Source: CAD feature listing. Evaluate the final solid. Frame: model axes, mm. Face numbers are marked on the shaded views. A direction names the side the tool comes from. Give positions to 0.01 mm unless a question says otherwise; leave off trailing zeros. Order: outer loops, then holes, each group sorted by start corner. A loop starts at its lowest first (then second) coordinate and runs counter-clockwise, first axis right, second up. Notation, with made-up numbers: (47.5, 32.25) - (94.5, 32.25) arc R29 cw to (94.5, 59.25) - close; hole circle Ø3 at (63, 76.5). An arc over 180 degrees is marked (long way). Answer as CSV lines item,"result".
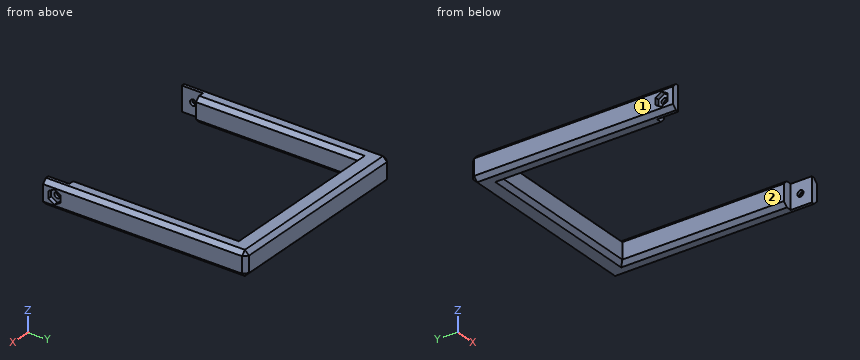
```python
from build123d import *

# Parameters (mm, degrees)
SKETCH1_W             = 3.5
SKETCH1_H             = 12
BOSS_EXTRUDE1_DEPTH   = 100
BOSS_EXTRUDE1_2_DEPTH = 100
SKETCH2_W             = 12
SKETCH2_H             = 10
BOSS_EXTRUDE2_DEPTH   = 90.08829946
SKETCH3_W             = 4.58560389
SKETCH3_H             = 12
BOSS_EXTRUDE3_DEPTH   = 79.6
CHAMFER6_SIZE         = 2
CUT_EXTRUDE1_DEPTH    = 2
CUT_EXTRUDE2_REACH    = 140.122
SKETCH5_R             = 1.5


with BuildPart() as part:
    # Sketch1 → Boss-Extrude1 (new body)
    with BuildSketch(Plane(origin=(0, 0, 0), x_dir=(1, 0, 0), z_dir=(0, 1, 0))):
        with Locations((-46.79414973, 0)):
            Rectangle(SKETCH1_W, SKETCH1_H)
    extrude(amount=BOSS_EXTRUDE1_DEPTH)



with BuildPart() as body_2:
    # Sketch1 → Boss-Extrude1 2 (new body)
    with BuildSketch(Plane(origin=(0, 0, 0), x_dir=(1, 0, 0), z_dir=(0, 1, 0))):
        with Locations((46.79414973, 0)):
            Rectangle(SKETCH1_W, SKETCH1_H)
    extrude(amount=BOSS_EXTRUDE1_2_DEPTH)


with BuildPart() as part_1:
    add(part.part)

    add(body_2.part)  # Boss-Extrude2 merges body 2
    # Sketch2 → Boss-Extrude2 (add)
    with BuildSketch(Plane(origin=(-45.04414973, 0, 0), x_dir=(0, 0, -1), z_dir=(1, 0, 0))):
        with Locations((0, 95)):
            Rectangle(SKETCH2_W, SKETCH2_H)
    extrude(amount=BOSS_EXTRUDE2_DEPTH)

    # Sketch3 → Boss-Extrude3 (add)
    with BuildSketch(Plane.XZ.offset(-90)):
        with Locations((-42.751347785, 0)):
            Rectangle(SKETCH3_W, SKETCH3_H)
        with Locations((42.751347785, 0)):
            Rectangle(SKETCH3_W, SKETCH3_H)
    extrude(amount=BOSS_EXTRUDE3_DEPTH)

    # Chamfer6
    chamfer6_edges = [part_1.edges().sort_by_distance(p)[0] for p in [
        (0, 100, 6),
        (48.54414973, 50, 6),
        (48.54414973, 50, -6),
        (48.54414973, 100, 0),
        (0, 100, -6),
        (-40.45854584, 50.2, -6),
        (-40.45854584, 50.2, 6),
        (0, 90, 6),
        (0, 90, -6),
        (40.45854584, 50.2, 6),
        (40.45854584, 50.2, -6),
        (-48.54414973, 50, 6),
        (-48.54414973, 50, -6),
        (-48.54414973, 100, 0),
    ]]
    chamfer(chamfer6_edges, length=CHAMFER6_SIZE)

    # Sketch4 → Cut-Extrude1 (cut)
    with BuildSketch(Plane(origin=(48.54414973, 0, 0), x_dir=(0, 0, -1), z_dir=(1, 0, 0))):
        Polygon((3.464101615, 5.6), (1.732050808, 8.6), (-1.732050808, 8.6), (-3.464101615, 5.6), (-1.732050808, 2.6), (1.732050808, 2.6), align=None)
    cut_extrude1 = extrude(amount=-CUT_EXTRUDE1_DEPTH, mode=Mode.SUBTRACT)

    # Mirror1: Cut-Extrude1 across plane
    add(cut_extrude1.mirror(Plane(origin=(0, 0, 0), x_dir=(0, 0, 1), z_dir=(1, 0, 0))), mode=Mode.SUBTRACT)

    # Cut-Extrude2: up to this face of the body (flat: up to its plane)
    cut_extrude2_end = Plane(part_1.part.faces().sort_by_distance((-46.54414973, 5.6, 0))[0])
    # Sketch5 → Cut-Extrude2 (cut, up to the picked face)
    with BuildSketch(Plane(origin=(46.54414973, 0, 0), x_dir=(0, 0, -1), z_dir=(1, 0, 0)), mode=Mode.PRIVATE) as cut_extrude2_sk1:
        with Locations((0, 5.6)):
            Circle(SKETCH5_R)
    cut_extrude2_tool1 = split(extrude(cut_extrude2_sk1.sketch, amount=-CUT_EXTRUDE2_REACH, mode=Mode.PRIVATE), bisect_by=cut_extrude2_end, keep=Keep.BOTH, mode=Mode.PRIVATE)
    add(cut_extrude2_tool1.solids().sort_by(Axis((46.54415, 5.6, 0), (-1, 0, 0)))[0], mode=Mode.SUBTRACT)


solid = part_1.part
```
(1) Cut plane B-B (y = 69). Return loops of the section in (x, z).
Completed:
outline,"(-48.54, -4) - (-46.54, -6) - (-42.46, -6) - (-40.46, -4) - (-40.46, 4) - (-42.46, 6) - (-46.54, 6) - (-48.54, 4) - close; (40.46, -4) - (42.46, -6) - (46.54, -6) - (48.54, -4) - (48.54, 4) - (46.54, 6) - (42.46, 6) - (40.46, 4) - close"
(2) Ray query, line 1 (Y direction, x = -45.9, z = 0); line 2 (X direction, y = 66, z = -1); line 3 (X direction, y = 8, z = -0.5). Return the intervals inside material, ascending. Write a range as from..to.
Completed:
line 1,"0..4.1, 7.1..100"
line 2,"-48.54..-40.46, 40.46..48.54"
line 3,"-46.54..-45.04, 45.04..46.54"
(3) Cut plane A-A (z = 0). Give the number of separate pieces and of enclosed holes in the cut face, then the cut area to 3 significant figures.
Completed:
separate pieces,"3"
enclosed holes,"0"
area,"2,290 mm²"
(4) Cut plane C-C (x = -37.5). Return loops of the section in (y, z), then the cut area to 3 significant figures.
Completed:
outline,"(90, -4) - (92, -6) - (98, -6) - (100, -4) - (100, 4) - (98, 6) - (92, 6) - (90, 4) - close"
area,"112 mm²"
(5) Contact query for flat-ended pins moving along their axis: pin 1 (3.5 mm diameter, centred on y = 5.6, z = 0, fed in from +X); pin 2 (2.5 mm diameter, centred on x = -42, z = 0, fed in from -Y); pin 3 (3 mm diameter, centred on x = -5, z = -0.5, fed in from -Y). Output: stop coordinate, or through.
Completed:
pin 1,"x = 46.54"
pin 2,"y = 10.4"
pin 3,"y = 90"
(6) Access query for the marked faces 1 and 2. Directions: +Z, -Z, +X, -X, +Y, -Y. A direction counts if a zero-diameter tool reaches every point of the face in a straight line with its end or side. Return the directions, or none.
Completed:
face 1,"+Z, -Z, -X, +Y, -Y"
face 2,"+Z, -Z, -Y"
